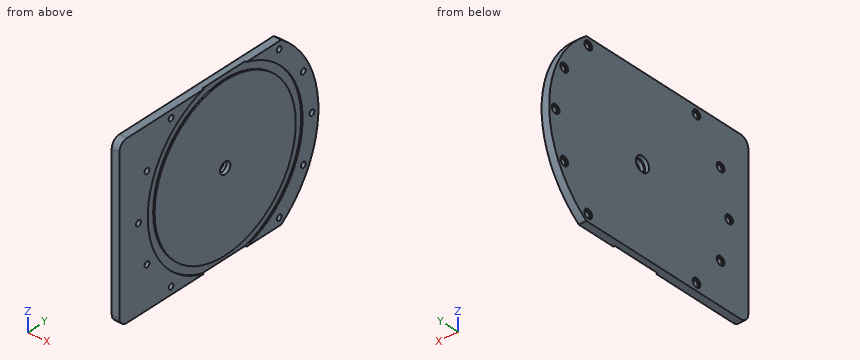
```python
from build123d import *

# Parameters (mm, degrees)
SKETCH1_R           = 5.08
BOSS_EXTRUDE1_DEPTH = 6.604
SKETCH2_R           = 6.477
CUT_EXTRUDE1_DEPTH  = 3.302
SKETCH3_R           = 75.946
SKETCH3_R_2         = 69.215
CUT_EXTRUDE2_DEPTH  = 1.27
SKETCH4_R           = 2.38125
CUT_EXTRUDE3_DEPTH  = 139.530727768
SKETCH5_R           = 3.77825
CUT_EXTRUDE4_DEPTH  = 1.27
SKETCH6_W           = 37.512644612
SKETCH6_H           = 125.02997604
SKETCH6_W_2         = 29.936636925
CUT_EXTRUDE6_DEPTH  = 139.530727768


with BuildPart() as part:
    # Sketch1 → Boss-Extrude1 (new body)
    with BuildSketch(Plane(origin=(0, 0, 0), x_dir=(0, 0, -1), z_dir=(1, 0, 0))):
        with BuildLine():
            Line((-65.405, -103.855072673), (65.405, -103.855072673))
            ThreePointArc((65.405, -103.855072673), (70.793153673, -101.623226346), (73.025, -96.235072673))
            Line((73.025, -96.235072673), (73.025, -69.997049759))
            ThreePointArc((73.025, -69.997049759), (74.696702219, -57.072253546), (79.601785714, -44.998103417))
            ThreePointArc((79.601785714, -44.998103417), (0, 91.44), (-79.601785714, -44.998103417))
            ThreePointArc((-79.601785714, -44.998103417), (-74.696702219, -57.072253546), (-73.025, -69.997049759))
            Line((-73.025, -69.997049759), (-73.025, -96.235072673))
            ThreePointArc((-73.025, -96.235072673), (-70.793153673, -101.623226346), (-65.405, -103.855072673))
        make_face()
        with Locations(Location((0, 0, 0), (0, 0, 180))):
            Circle(SKETCH1_R, mode=Mode.SUBTRACT)
    extrude(amount=BOSS_EXTRUDE1_DEPTH)

    # Sketch2 → Cut-Extrude1 (cut)
    with BuildSketch(Plane(origin=(0, 0, 0), x_dir=(0, 0, -1), z_dir=(1, 0, 0))):
        with Locations(Location((0, 0, 0), (0, 0, 180))):
            Circle(SKETCH2_R)
    extrude(amount=CUT_EXTRUDE1_DEPTH, mode=Mode.SUBTRACT)

    # Sketch3 → Cut-Extrude2 (cut)
    with BuildSketch(Plane(origin=(6.604, 0, 0), x_dir=(0, 0, -1), z_dir=(1, 0, 0))):
        Circle(SKETCH3_R)
        Circle(SKETCH3_R_2, mode=Mode.SUBTRACT)
    extrude(amount=-CUT_EXTRUDE2_DEPTH, mode=Mode.SUBTRACT)

    # Sketch4 → Cut-Extrude3 (cut, through all)
    with BuildSketch(Plane.ZY):
        with Locations((-82.956616048, 18.93430627)):
            Circle(SKETCH4_R)
        with Locations((0, 85.09)):
            Circle(SKETCH4_R)
        with Locations((-66.526040843, 53.05274724)):
            Circle(SKETCH4_R)
        with Locations((36.919167362, 76.66344097)):
            Circle(SKETCH4_R)
        with Locations((66.526040843, 53.05274724)):
            Circle(SKETCH4_R)
        with Locations((82.956616048, 18.93430627)):
            Circle(SKETCH4_R)
        with Locations((82.956616048, -18.93430627)):
            Circle(SKETCH4_R)
        with Locations((66.526040843, -53.05274724)):
            Circle(SKETCH4_R)
        with Locations((36.919167362, -76.66344097)):
            Circle(SKETCH4_R)
        with Locations((0, -85.09)):
            Circle(SKETCH4_R)
        with Locations((-36.919167361, -76.66344097)):
            Circle(SKETCH4_R)
        with Locations((-66.526040843, -53.05274724)):
            Circle(SKETCH4_R)
        with Locations((-82.956616048, -18.93430627)):
            Circle(SKETCH4_R)
        with Locations((-36.919167362, 76.66344097)):
            Circle(SKETCH4_R)
    extrude(amount=-CUT_EXTRUDE3_DEPTH, mode=Mode.SUBTRACT)

    # Sketch5 → Cut-Extrude4 (cut)
    with BuildSketch(Plane.ZY):
        with Locations((0, 85.09)):
            Circle(SKETCH5_R)
        with Locations((-82.956616048, 18.93430627)):
            Circle(SKETCH5_R)
        with Locations((-66.526040843, 53.05274724)):
            Circle(SKETCH5_R)
        with Locations((36.919167362, 76.66344097)):
            Circle(SKETCH5_R)
        with Locations((-36.919167362, 76.66344097)):
            Circle(SKETCH5_R)
        with Locations((66.526040843, 53.05274724)):
            Circle(SKETCH5_R)
        with Locations((82.956616048, 18.93430627)):
            Circle(SKETCH5_R)
        with Locations((82.956616048, -18.93430627)):
            Circle(SKETCH5_R)
        with Locations((66.526040843, -53.05274724)):
            Circle(SKETCH5_R)
        with Locations((36.919167362, -76.66344097)):
            Circle(SKETCH5_R)
        with Locations((0, -85.09)):
            Circle(SKETCH5_R)
        with Locations((-36.919167362, -76.66344097)):
            Circle(SKETCH5_R)
        with Locations((-66.526040843, -53.05274724)):
            Circle(SKETCH5_R)
        with Locations((-82.956616048, -18.93430627)):
            Circle(SKETCH5_R)
    extrude(amount=-CUT_EXTRUDE4_DEPTH, mode=Mode.SUBTRACT)

    # Sketch6 → Cut-Extrude6 (cut, through all)
    with BuildSketch(Plane(origin=(6.604, 0, 0), x_dir=(0, 0, -1), z_dir=(1, 0, 0))):
        with Locations((-91.781322306, -7.482061739)):
            Rectangle(SKETCH6_W, SKETCH6_H)
        with Locations((87.993318463, -7.482061739)):
            Rectangle(SKETCH6_W_2, SKETCH6_H)
    extrude(amount=-CUT_EXTRUDE6_DEPTH, mode=Mode.SUBTRACT)


solid = part.part
```
Verification items for the finished model (mm, model axes). Give positions to 0.01 mm unless a question says otherwise; leave off trailing zeros. Loops run counter-clockwise (first coordinate to the right, second up) from the corner with the lowest first, then second, coordinate; pieces in that order, holes last. Notation, with made-up numbers: M 18,2 L 41,2 A26 ccw 41,41 Z; hole C 5,-6.5 d6. An arc over 180 degrees is marked long. Return JSON: item names as keys, results as strings.
1) Section check C-C, the plane y = 0. Enter the section's corners in (x, z) (3 decimals), and give its area (3 significant figures).
Findings:
{"outline": "M 0,-73.025 L 5.334,-73.025 L 5.334,-69.215 L 6.604,-69.215 L 6.604,-5.08 L 3.302,-5.08 L 3.302,-6.477 L 0,-6.477 Z; M 0,6.477 L 3.302,6.477 L 3.302,5.08 L 6.604,5.08 L 6.604,69.215 L 5.334,69.215 L 5.334,73.025 L 0,73.025 Z", "area": "879 mm2"}
2) Material ranges on L1, parallel to Y at x = 1.7, z = 0; L2, parallel to Z at x = 6, y = -60 (3 decimals); L3, parallel to Z at x = 5.75, y = 39.5 (3 decimals), recorded low to high. Write a range as [from, to].
Findings:
{"L1": "y = [-103.86, -87.47], [-82.71, -6.48], [6.48, 82.71], [87.47, 91.44]", "L2": "z = [-73.025, -46.56], [-34.507, 34.507], [46.56, 73.025]", "L3": "z = [-73.025, -64.866], [-56.837, 56.837], [64.866, 73.025]"}
3) Section check D-D, the plane z = 60.5. Enter the section's corners in (x, y), and give its area (3 significant figures).
Findings:
{"outline": "M 0,-103.86 L 6.6,-103.86 L 6.6,-45.91 L 5.33,-45.91 L 5.33,-33.62 L 6.6,-33.62 L 6.6,33.62 L 5.33,33.62 L 5.33,45.91 L 6.6,45.91 L 6.6,68.56 L 0,68.56 Z", "area": "1,110 mm2"}
4) Section check B-B, the plane z = 0. Count the separate pieces of the cut face and the enclosed holes in it, and give its area (3 significant figures).
Findings:
{"separate pieces": "4", "enclosed holes": "0", "area": "1,130 mm2"}
5) Section check A-A, the plane y = -85.09. Enter the section's corners in (x, z) (3 decimals).
Findings:
{"outline": "M 0,-73.025 L 6.604,-73.025 L 6.604,-2.381 L 1.27,-2.381 L 1.27,-3.778 L 0,-3.778 Z; M 0,3.778 L 1.27,3.778 L 1.27,2.381 L 6.604,2.381 L 6.604,73.025 L 0,73.025 Z"}
6) Gauge pin test, flat ends, axial feed: P1, Ø8.5, axis at y = 53.05, z = -66.53, coming from the -X side; P2, Ø1, axis at x = 2, z = 30.5, coming from the +Y side; P3, Ø2.5, axis at y = -83.5, z = -0.5, coming from the -X side. Record the tip position at first contact, or that the pin passes through.
Findings:
{"P1": "stops at x = 0", "P2": "stops at y = 86.38", "P3": "stops at x = 1.27"}
